```python
from build123d import *

# Parameters (mm, degrees)
F1_DEPTH  = 8.5
F2_R      = 3
F3_DEPTH  = 5
F2_R_2    = 4
F4_DEPTH  = 4
F5_R      = 3
F6_DEPTH  = 5
F5_R_2    = 4
F7_DEPTH  = 4
F9_D      = 3
F10_D     = 3
F10_DEPTH = 10
F10_TIP   = 0.9012909285


with BuildPart() as f1:
    # F0 (on Top) → F1 (new body, symmetric)
    with BuildSketch(Plane.XY):
        Polygon((19, 13.5), (-11, 13.5), (-11, 8.5), (0, 8.5), (0, -8.5), (-11, -8.5), (-11, -13.5), (19, -13.5), align=None)
    extrude(amount=F1_DEPTH, both=True)

    # F2 (on face) → F3 (cut, through all)
    with BuildSketch(Plane.XZ.offset(13.5)):
        with Locations((-6.5, 0)):
            Circle(F2_R)
    extrude(amount=-F3_DEPTH, mode=Mode.SUBTRACT)

    # F2 (on face) → F4 (cut)
    with BuildSketch(Plane.XZ.offset(13.5)):
        with Locations((-6.5, 0)):
            Circle(F2_R_2)
        with Locations((-6.5, 0)):
            Circle(F2_R, mode=Mode.SUBTRACT)
    extrude(amount=-F4_DEPTH, mode=Mode.SUBTRACT)

    # F5 (on face) → F6 (cut, through all)
    with BuildSketch(Plane(origin=(0, 13.5, 0), x_dir=(-1, 0, 0), z_dir=(0, 1, 0))):
        with Locations((6.5, 0)):
            Circle(F5_R)
    extrude(amount=-F6_DEPTH, mode=Mode.SUBTRACT)

    # F5 (on face) → F7 (cut)
    with BuildSketch(Plane(origin=(0, 13.5, 0), x_dir=(-1, 0, 0), z_dir=(0, 1, 0))):
        with Locations((6.5, 0)):
            Circle(F5_R_2)
        with Locations((6.5, 0)):
            Circle(F5_R, mode=Mode.SUBTRACT)
    extrude(amount=-F7_DEPTH, mode=Mode.SUBTRACT)

    # F9 (through all)
    with Locations(Plane.YZ.offset(19)):
        with Locations((-11, 6), (-11, -6), (11, -6), (11, 6)):
            Hole(F9_D / 2)

    # F10
    with Locations(Plane.XZ.offset(13.5)):
        with Locations((12, 0)):
            Hole(F10_D / 2, depth=F10_DEPTH)
            with Locations((0, 0, -(F10_DEPTH + F10_TIP / 2))):  # 118° drill point
                Cone(0, F10_D / 2, F10_TIP, mode=Mode.SUBTRACT)


solid = f1.part
```
Source: CAD feature listing. Evaluate the final solid. Frame: model axes, mm. A direction names the side the tool comes from. Round coordinates to 2 decimals unless told otherwise and drop trailing zeros. Loops run counter-clockwise (first coordinate to the right, second up) from the corner with the lowest first, then second, coordinate; pieces in that order, holes last. Notation, with made-up numbers: M 32,86 L 50,86 A12 ccw 50,108 Z; hole C 29.25,-14.5 d6. An arc over 180 degrees is marked long. Use a Markdown table: item, result. Add a question column.
1. Section query B-B on z = 6. Return the cut outline in (x, y).
2. Contact query for flat-ended pins moving along their axis: P1, Ø1, axis at y = 5, z = -1.5, coming from the -X side; P2, Ø7, axis at x = -6.5, z = 0, coming from the -Y side; P3, Ø5, axis at x = -6.5, z = 0, coming from the -Y side; P4, Ø6.5, axis at x = -6.5, z = 0.5, coming from the +Y side. Output: stop coordinate, or through.
3. Section query A-A on y = -11. Return the cut outline in (x, z), then the cut area to 3 significant figures.
4. Section query C-C on y = 11. Return the cut outline in (x, z), then the cut area to 3 significant figures.
5. Section query D-D on z = -7. Return the cut outline in (x, y).
6. Line query: line 1 (Z direction, x = 6, y = 11); line 2 (Z direction, x = -6.5, y = 11.6); line 3 (Z direction, x = 12, y = -9.25). Output: solid intervals per line, ascending.
7. Reachability of faces 5 (the flat face through (-3, 8.5, 0)), 6 (the cylindrical face through (-7.367, -11.528, -3.905)), 7 (the cylindrical face through (-9.27, 9.01, -1.15)) from +Z, -Z, +X, -X, +Y, -Y: full face, straight path, thin tool, end or side. Return the list, or none.
8. Mould query, pull axis Y, two halves, no side actions, for faces 1 (the flat face through (-4, -8.5, 2)), 2 (the cylindrical face through (-5.633, 11.528, -3.905)), 3 (the cylindrical face through (3.79, -9.5, 6.07)), 4 (the flat face through (-8, 9.5, 3)). Classes: pulls with the +Y half, pulls with the -Y half, needs draft (parallel to the pull), parting line crosses it, or undercut.
Reported:
| question | item | result |
|---|---|---|
| 1 | outline | M -11,-13.5 L 19,-13.5 L 19,-12.5 L -11,-12.5 Z; M -11,-9.5 L 19,-9.5 L 19,9.5 L -11,9.5 L -11,8.5 L 0,8.5 L 0,-8.5 L -11,-8.5 Z; M -11,12.5 L 19,12.5 L 19,13.5 L -11,13.5 Z |
| 2 | P1 | stops at x = 0 |
| 2 | P2 | stops at y = -9.5 |
| 2 | P3 | passes through |
| 2 | P4 | stops at y = 9.5 |
| 3 | outline | M -11,-8.5 L 19,-8.5 L 19,-7.5 L -11,-7.5 Z; M -11,-4.5 L 19,-4.5 L 19,4.5 L -11,4.5 Z; M -11,7.5 L 19,7.5 L 19,8.5 L -11,8.5 Z; hole C -6.5,0 d8; hole C 12,0 d3 |
| 3 | area | 273 mm² |
| 4 | outline | M -11,-8.5 L 19,-8.5 L 19,-7.5 L -11,-7.5 Z; M -11,-4.5 L 19,-4.5 L 19,4.5 L -11,4.5 Z; M -11,7.5 L 19,7.5 L 19,8.5 L -11,8.5 Z; hole C -6.5,0 d8 |
| 4 | area | 280 mm² |
| 5 | outline | M -11,-13.5 L 19,-13.5 L 19,-12.12 L -11,-12.12 Z; M -11,-9.88 L 19,-9.88 L 19,9.88 L -11,9.88 L -11,8.5 L 0,8.5 L 0,-8.5 L -11,-8.5 Z; M -11,12.12 L 19,12.12 L 19,13.5 L -11,13.5 Z |
| 6 | line 1 | z = -8.5 to -7.5, -4.5 to 4.5, 7.5 to 8.5 |
| 6 | line 2 | z = -8.5 to -7.37, -4.63 to -4, 4 to 4.63, 7.37 to 8.5 |
| 6 | line 3 | z = -8.5 to -1.5, 1.5 to 8.5 |
| 7 | face 5 | +Z, -Z, -X |
| 7 | face 6 | -Y |
| 7 | face 7 | +Y, -Y |
| 8 | face 1 | undercut |
| 8 | face 2 | needs draft |
| 8 | face 3 | undercut |
| 8 | face 4 | pulls with the +Y half |
